Input: part model. Units: mm. Frame: model coordinates. A direction names the side the tool comes from. Give positions to 0.01 mm unless a question says otherwise; leave off trailing zeros. Write each loop counter-clockwise with the first axis right and the second up, starting at its lowest first coordinate (ties: lowest second). Pieces come first, ordered by that corner, then holes. Notation, with made-up numbers: (69.5, -0.5) - (118.5, -0.5) arc R29 cw to (118.5, 26.5) - close; hole circle Ø3 at (30, 27). An arc over 180 degrees is marked (long way). Use a Markdown table: item, result. Add a question column.
1. Set-up query: faces 1 (the flat face through (30, 3, 2)), 2 (the cylindrical face through (-37, 16, 1)), 3 (the flat face through (29, 25, 1)). Return all of +Z, -Z, +X, -X, +Y, -Y with unobstructed straight access to the full face (end or side cutting, diameter ignored); none if empty.
2. Section query A-A, the plane y = 15. Return loops of the section in (x, z), plus the area to 3 significant figures.
3. Pin query (flat end, axial travel): pin 1 (0.9 mm diameter, centred on x = 26.5, z = 1.5, fed in from +Y); pin 2 (8 mm diameter, centred on x = -3, y = 14.5, fed in from -Z); pin 3 (1.5 mm diameter, centred on x = -36, z = 2, fed in from -Y); pin 4 (1.5 mm diameter, centred on y = 4.5, z = 2, fed in from +X). Return the tip coordinate at first contact, or that it passes through.
4. Section query D-D, the plane x = 0. Return loops of the section in (y, z), plus the area to 3 significant figures.
5. Mould query, pull axis Y, two halves, no side actions, for faces 4 (the flat face through (-30, 3, 2)), 5 (the cylindrical face through (37, 14, 1)), 6 (the flat face through (-28, 25, 1)), 7 (the cylindrical face through (10, 46, 1)). Classes: released by +Y, released by -Y, zero draft, split by the parting line, or undercut.
6. Section query B-B, the plane x = -37. Return loops of the section in (y, z), plus the area to 3 significant figures.
7. Section query C-C, the plane y = 40. Return loops of the section in (x, z).
8. Material intervals for probe 1 along Y at (x, z) = (0, 1); probe 2 along Y at (x, z) = (-10, 0.7); probe 3 along X at (y, z) = (19.5, 2.7), sorted ascending.
```python
from build123d import *

# Parameters (mm, degrees)
ESQUISSE1_R             = 13
BOSS_EXTRU_1_DEPTH      = 12
BOSS_EXTRU_2_START      = -12
ESQUISSE2_R             = 13
ESQUISSE2_R_2           = 5.5
BOSS_EXTRU_2_DEPTH      = 3
ESQUISSE4_R             = 8
ENL_V_MAT_EXTRU_2_DEPTH = 6
ESQUISSE5_R             = 3
ENL_V_MAT_EXTRU_3_DEPTH = 69.271516755
ESQUISSE6_W             = 10
ESQUISSE6_H             = 6
ENL_V_MAT_EXTRU_4_DEPTH = 12
CHANFREIN1_SIZE         = 5
ESQUISSE7_R             = 1
ENL_V_MAT_EXTRU_5_DEPTH = 12
ESQUISSE8_W             = 80
ESQUISSE8_H             = 9
ENL_V_MAT_EXTRU_6_DEPTH = 70.057946682


with BuildPart() as part:
    # Esquisse1 → Boss.-Extru.1 (new body)
    with BuildSketch(Plane.XY):
        Polygon((-40, 0), (40, 0), (40, 25), (17, 25), (17, 55), (-17, 55), (-17, 25), (-40, 25), align=None)
        with Locations((0, 40)):
            Circle(ESQUISSE1_R, mode=Mode.SUBTRACT)
    extrude(amount=BOSS_EXTRU_1_DEPTH)

    # Esquisse2 → Boss.-Extru.2 (add)
    with BuildSketch(Plane.XY.offset(12).offset(BOSS_EXTRU_2_START)):
        with Locations((0, 40)):
            Circle(ESQUISSE2_R)
        with Locations((0, 40)):
            Circle(ESQUISSE2_R_2, mode=Mode.SUBTRACT)
    extrude(amount=BOSS_EXTRU_2_DEPTH)

    # Esquisse4 → Enlèv. mat.-Extru.2 (cut)
    with BuildSketch(Plane(origin=(0, 0, 0), x_dir=(-1, 0, 0), z_dir=(0, 0, -1))):
        with Locations((-25, 15)):
            Circle(ESQUISSE4_R)
        with Locations(Location((25, 15, 0), (0, 0, 180))):
            Circle(ESQUISSE4_R)
    extrude(amount=-ENL_V_MAT_EXTRU_2_DEPTH, mode=Mode.SUBTRACT)

    # Esquisse5 → Enlèv. mat.-Extru.3 (cut, through all)
    with BuildSketch(Plane(origin=(0, 0, 6), x_dir=(-1, 0, 0), z_dir=(0, 0, -1))):
        with Locations((-25, 15)):
            Circle(ESQUISSE5_R)
        with Locations(Location((25, 15, 0), (0, 0, 180))):
            Circle(ESQUISSE5_R)
    extrude(amount=-ENL_V_MAT_EXTRU_3_DEPTH, mode=Mode.SUBTRACT)

    # Esquisse6 → Enlèv. mat.-Extru.4 (cut)
    with BuildSketch(Plane.XY.offset(12)):
        with Locations((35, 3)):
            Rectangle(ESQUISSE6_W, ESQUISSE6_H)
        with Locations((-35, 3)):
            Rectangle(ESQUISSE6_W, ESQUISSE6_H)
    extrude(amount=-ENL_V_MAT_EXTRU_4_DEPTH, mode=Mode.SUBTRACT)

    # Chanfrein1
    chanfrein1_edges = [part.edges().sort_by_distance(p)[0] for p in [
        (-17, 55, 6),
        (17, 55, 6),
        (17, 25, 6),
        (40, 25, 6),
        (-40, 25, 6),
        (-17, 25, 6),
    ]]
    chamfer(chanfrein1_edges, length=CHANFREIN1_SIZE)

    # Esquisse7 → Enlèv. mat.-Extru.5 (cut)
    with BuildSketch(Plane(origin=(0, 0, 0), x_dir=(-1, 0, 0), z_dir=(0, 0, -1))):
        with Locations((-10, 45)):
            Circle(ESQUISSE7_R)
        with Locations(Location((10, 45, 0), (0, 0, 180))):
            Circle(ESQUISSE7_R)
        with Locations((-37, 15)):
            Circle(ESQUISSE7_R)
        with Locations(Location((37, 15, 0), (0, 0, 180))):
            Circle(ESQUISSE7_R)
        with Locations((0, 15)):
            Circle(ESQUISSE7_R)
    extrude(amount=-ENL_V_MAT_EXTRU_5_DEPTH, mode=Mode.SUBTRACT)

    # Esquisse8 → Enlèv. mat.-Extru.6 (cut, through all)
    with BuildSketch(Plane(origin=(0, 55, 0), x_dir=(1, 0, 0), z_dir=(0, 1, 0))):
        with Locations((0, -7.5)):
            Rectangle(ESQUISSE8_W, ESQUISSE8_H)
    extrude(amount=-ENL_V_MAT_EXTRU_6_DEPTH, mode=Mode.SUBTRACT)


solid = part.part
```
Result sheet:
| question | item | result |
|---|---|---|
| 1 | face 1 | +Z, -Z, +X, -Y |
| 1 | face 2 | +Z, -Z |
| 1 | face 3 | +Z, -Z, +X, +Y |
| 2 | outline | (-40, 0) - (-38, 0) - (-38, 3) - (-40, 3) - close; (-36, 0) - (-33, 0) - (-33, 3) - (-36, 3) - close; (-17, 0) - (-1, 0) - (-1, 3) - (-17, 3) - close; (1, 0) - (17, 0) - (17, 3) - (1, 3) - close; (33, 0) - (36, 0) - (36, 3) - (33, 3) - close; (38, 0) - (40, 0) - (40, 3) - (38, 3) - close |
| 2 | area | 126 mm² |
| 3 | pin 1 | stops at y = 25 |
| 3 | pin 2 | stops at z = 0 |
| 3 | pin 3 | stops at y = 6 |
| 3 | pin 4 | stops at x = 30 |
| 4 | outline | (0, 0) - (14, 0) - (14, 3) - (0, 3) - close; (16, 0) - (34.5, 0) - (34.5, 3) - (16, 3) - close; (45.5, 0) - (55, 0) - (55, 3) - (45.5, 3) - close |
| 4 | area | 126 mm² |
| 5 | face 4 | zero draft |
| 5 | face 5 | undercut |
| 5 | face 6 | released by +Y |
| 5 | face 7 | undercut |
| 6 | outline | (6, 0) - (14, 0) - (14, 3) - (6, 3) - close; (16, 0) - (23, 0) - (23, 3) - (16, 3) - close |
| 6 | area | 45.0 mm² |
| 7 | outline | (-17, 0) - (-5.5, 0) - (-5.5, 3) - (-17, 3) - close; (5.5, 0) - (17, 0) - (17, 3) - (5.5, 3) - close |
| 8 | probe 1 | y = 0 to 14, 16 to 34.5, 45.5 to 55 |
| 8 | probe 2 | y = 0 to 44, 46 to 55 |
| 8 | probe 3 | x = -40 to -31.61, -18.39 to 18.39, 31.61 to 40 |
